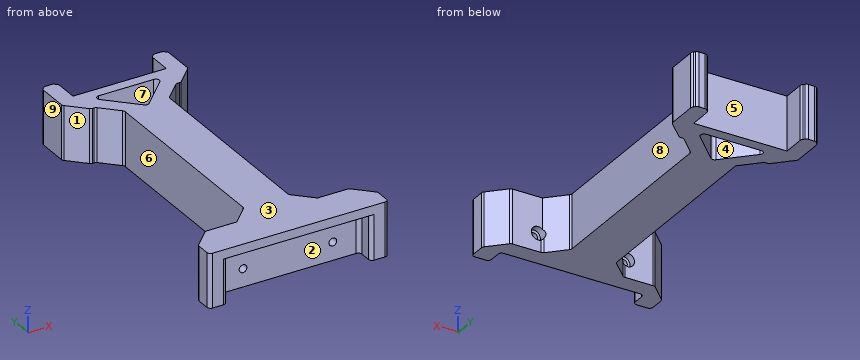
from build123d import *

# Parameters (mm, degrees)
EXTRUDE_1_DEPTH     = 30
SKETCH_3_W          = 52
SKETCH_3_H          = 30
CUT_EXTRUDE_1_DEPTH = 190.208879284
SKETCH_4_W          = 80
SKETCH_4_H          = 20
CUT_EXTRUDE_2_DEPTH = 25
SKETCH_5_R          = 2.15
CUT_EXTRUDE_3_DEPTH = 171.293863659
SKETCH_6_R          = 3.7
CUT_EXTRUDE_4_DEPTH = 4
CHAMFER_1_SIZE      = 10
CHAMFER_2_SIZE      = 2
FILLET_1_R          = 2
CUT_EXTRUDE_5_DEPTH = 190.208879284
FILLET_2_R          = 2


with BuildPart() as part:
    # 草图2 → 凸台-拉伸1 (new body)
    with BuildSketch(Plane.XY):
        Polygon((-35, 180), (35, 180), (35, 150), (12.5, 150), (12.5, 20), (50, 20), (50, 0), (-50, 0), (-50, 20), (-12.5, 20), (-12.5, 150), (-35, 150), align=None)
    extrude(amount=EXTRUDE_1_DEPTH)

    # 草图3 → 切除-拉伸1 (cut, through all)
    with BuildSketch(Plane(origin=(0, 0, 30), x_dir=(-1, 0, 0), z_dir=(0, 0, -1))):
        with Locations((0, 180)):
            Rectangle(SKETCH_3_W, SKETCH_3_H)
    extrude(amount=CUT_EXTRUDE_1_DEPTH, mode=Mode.SUBTRACT)

    # 草图4 → 切除-拉伸2 (cut)
    with BuildSketch(Plane(origin=(0, 0, 0), x_dir=(-1, 0, 0), z_dir=(0, 0, -1))):
        Rectangle(SKETCH_4_W, SKETCH_4_H)
    extrude(amount=-CUT_EXTRUDE_2_DEPTH, mode=Mode.SUBTRACT)

    # 草图5 → 切除-拉伸3 (cut, through all)
    with BuildSketch(Plane(origin=(0, 20, 0), x_dir=(1, 0, 0), z_dir=(0, 1, 0))):
        with Locations(Location((-25, -10, 0), (0, 0, 180))):
            Circle(SKETCH_5_R)
        with Locations(Location((25, -10, 0), (0, 0, 180))):
            Circle(SKETCH_5_R)
    extrude(amount=-CUT_EXTRUDE_3_DEPTH, mode=Mode.SUBTRACT)

    # 草图6 → 切除-拉伸4 (cut)
    with BuildSketch(Plane(origin=(0, 20, 0), x_dir=(1, 0, 0), z_dir=(0, 1, 0))):
        with Locations(Location((25, -10, 0), (0, 0, 180))):
            Circle(SKETCH_6_R)
        with Locations(Location((-25, -10, 0), (0, 0, 180))):
            Circle(SKETCH_6_R)
    extrude(amount=-CUT_EXTRUDE_4_DEPTH, mode=Mode.SUBTRACT)

    # 倒角1
    # the kernel refuses this chamfer: 10 mm, written as the material it adds along each edge
    with BuildSketch(Plane(origin=(12.5, 150, 0), x_dir=(-0.027495876610586452, -0.9996219169112968, 0), z_dir=(0, 0, 1)), Plane(origin=(-12.5, 150, 0), x_dir=(-0.9996219169112968, 0.0274958766105877, 0), z_dir=(0, 0, 1))) as chamfer_1_piece_1:
        Polygon((CHAMFER_1_SIZE * 0.999621916911, CHAMFER_1_SIZE * 0.0274958766106), (-CHAMFER_1_SIZE * 0.0274958766106, CHAMFER_1_SIZE * 0.999621916911), (0, 0), align=None)
    extrude(amount=30)
    with BuildSketch(Plane(origin=(12.5, 20, 0), x_dir=(0.9996219169112968, -0.027495876610586313, 0), z_dir=(0, 0, 1))) as chamfer_1_piece_2_section:
        Polygon((CHAMFER_1_SIZE * 0.999621916911, CHAMFER_1_SIZE * 0.0274958766106), (-CHAMFER_1_SIZE * 0.0274958766106, CHAMFER_1_SIZE * 0.999621916911), (0, 0), align=None)
    chamfer_1_piece_2 = extrude(amount=30, mode=Mode.PRIVATE)
    chamfer_1_piece_2 = chamfer_1_piece_2 - Plane(origin=(25, 23.307134121, 10), x_dir=(-1, 0, 0), z_dir=(0, 1, 0)) * Cylinder(3.7, 100, mode=Mode.PRIVATE)
    add(chamfer_1_piece_2)
    with BuildSketch(Plane(origin=(-12.5, 20, 0), x_dir=(0.027495876610586147, 0.9996219169112968, 0), z_dir=(0, 0, 1))) as chamfer_1_piece_3_section:
        Polygon((CHAMFER_1_SIZE * 0.999621916911, CHAMFER_1_SIZE * 0.0274958766106), (-CHAMFER_1_SIZE * 0.0274958766106, CHAMFER_1_SIZE * 0.999621916911), (0, 0), align=None)
    chamfer_1_piece_3 = extrude(amount=30, mode=Mode.PRIVATE)
    chamfer_1_piece_3 = chamfer_1_piece_3 - Plane(origin=(-25, 23.30713415, 10), x_dir=(-1, 0, 0), z_dir=(0, 1, 0)) * Cylinder(3.7, 100, mode=Mode.PRIVATE)
    add(chamfer_1_piece_3)
    # the kernel refuses this chamfer: 10 mm, written as the material it takes off along each edge
    with BuildSketch(Plane(origin=(35, 150, -25.71682988), x_dir=(-0.9996219169112968, -0.0274958766105877, 0), z_dir=(0, 0, 1)), Plane(origin=(-35, 150, -25.71682988), x_dir=(-0.027495876610586282, 0.9996219169112968, 0), z_dir=(0, 0, 1))) as chamfer_1_2_piece_1:
        Polygon((CHAMFER_1_SIZE * 0.999621916911, -CHAMFER_1_SIZE * 0.0274958766106), (-CHAMFER_1_SIZE * 0.0274958766106, -CHAMFER_1_SIZE * 0.999621916911), (0, 0), align=None)
    extrude(amount=81.433659759, mode=Mode.SUBTRACT)
    with BuildSketch(Plane(origin=(50, 20, -25.71682988), x_dir=(-0.9996219169112968, 0.027495876610586317, 0), z_dir=(0, 0, 1)), Plane(origin=(-50, 20, -25.71682988), x_dir=(-0.027495876610585626, -0.9996219169112968, 0), z_dir=(0, 0, 1))) as chamfer_1_2_piece_2:
        Polygon((CHAMFER_1_SIZE * 0.999621916911, CHAMFER_1_SIZE * 0.0274958766106), (-CHAMFER_1_SIZE * 0.0274958766106, CHAMFER_1_SIZE * 0.999621916911), (0, 0), align=None)
    extrude(amount=81.433659759, mode=Mode.SUBTRACT)

    # 倒角2
    chamfer_2_edges = [part.edges().sort_by_distance(p)[0] for p in [
        (-35, 180, 15),
        (35, 180, 15),
        (26, 180, 15),
        (-26, 180, 15),
    ]]
    chamfer(chamfer_2_edges, length=CHAMFER_2_SIZE)

    # 圆角1
    fillet_1_edges = [part.edges().sort_by_distance(p)[0] for p in [
        (-35, 160, 15),
        (-25, 150, 15),
        (-22.5, 150, 15),
        (-12.5, 140, 15),
        (-12.5, 30, 15),
        (-22.5, 20, 3.63618183),
        (-40, 20, 15),
        (-50, 10, 15),
        (-50, 0, 15),
        (-40, 0, 12.5),
        (-40, 10, 12.5),
        (40, 10, 12.5),
        (40, 0, 12.5),
        (50, 0, 15),
        (50, 10, 15),
        (40, 20, 15),
        (22.5, 20, 3.63618183),
        (12.5, 30, 15),
        (22.5, 150, 15),
        (25, 150, 15),
        (35, 160, 15),
        (35, 178, 15),
        (33, 180, 15),
        (28, 180, 15),
        (26, 178, 15),
        (-26, 178, 15),
        (-28, 180, 15),
        (-33, 180, 15),
        (-35, 178, 15),
        (12.5, 140, 15),
    ]]
    fillet(fillet_1_edges, radius=FILLET_1_R)

    # 草图7 → 切除-拉伸5 (cut, through all)
    with BuildSketch(Plane(origin=(0, 0, 0), x_dir=(-1, 0, 0), z_dir=(0, 0, -1))):
        Polygon((-20.186291501, 159), (0, 138.813708499), (20.186291501, 159), align=None)
    extrude(amount=-CUT_EXTRUDE_5_DEPTH, mode=Mode.SUBTRACT)

    # 圆角2
    fillet_2_edges = [part.edges().sort_by_distance(p)[0] for p in [
        (20.186291501, 159, 15),
        (-20.186291501, 159, 15),
        (0, 138.813708499, 15),
    ]]
    fillet(fillet_2_edges, radius=FILLET_2_R)


solid = part.part
Build history of the part. All positions in model axes, mm. Face numbers are marked on the shaded views. A direction names the side the tool comes from. Round coordinates to 2 decimals unless told otherwise and drop trailing zeros. Loops run counter-clockwise (first coordinate to the right, second up) from the corner with the lowest first, then second, coordinate; pieces in that order, holes last. Notation, with made-up numbers: (62, 60.25) -> (119, 60.25) arc R6 cw to (119, 64.25) -> close; hole circle Ø5 at (59.5, -6.75). An arc over 180 degrees is marked (long way). One line per item, written item: value. Start each with the question number.
Q1. Cut at B-B on y = 54. List the corners of the cut face in (x, z).
Q2. Probe line 1 along Z through (x, y) = (-25, 13.5); line 2 along Z through (x, y) = (25, 19.55); line 3 along Y through (x, z) = (13, 19.5). List the from-to ranges inside material, lowest first.
Q3. Two-plate mould, pull along X, no slides. Class the marked faces 1, 2, 3 and 4: released by +X, released by -X, zero draft, split by the parting line, or undercut.
Q4. Cut at A-A on z = 10. Count the separate pieces of the cut face and the enclosed holes in it, plus the area to 3 significant figures.
Q5. Drop flat-ended pins along their axis: pin 1 Ø3 at (y, z) = (44.5, 14.5) entering from -X; pin 2 Ø1.5 at (x, z) = (-13, 10) entering from -Y; pin 3 Ø8 at (x, z) = (24.5, 10) entering from +Y. Give the stop position or say it passes through.
Q6. 3-axis set-ups, long thin cutter, end or side, ignore diameter. For the marked faces 5, 6, 7, 8 and 9: which of +Z, -Z, +X, -X, +Y, -Y reach the whole face in a straight line?
Computed:
1. outline: (-12.5, 0) -> (12.5, 0) -> (12.5, 30) -> (-12.5, 30) -> close
2. line 1: 0 to 7.85, 12.15 to 30
2. line 2: 0 to 6.3, 13.7 to 30
2. line 3: 10 to 29.51, 140.49 to 151.81, 159 to 165
3. face 1: released by -X
3. face 2: undercut
3. face 3: zero draft
3. face 4: undercut
4. separate pieces: 3
4. enclosed holes: 1
4. area: 5,250 mm²
5. pin 1: x = -12.5
5. pin 2: y = 10
5. pin 3: y = 179.97
6. face 5: +Z, -Z, +Y
6. face 6: +Z, -Z, -X
6. face 7: +Z, -Z
6. face 8: +Z, -Z, +X
6. face 9: +Z, -Z, -X, +Y
